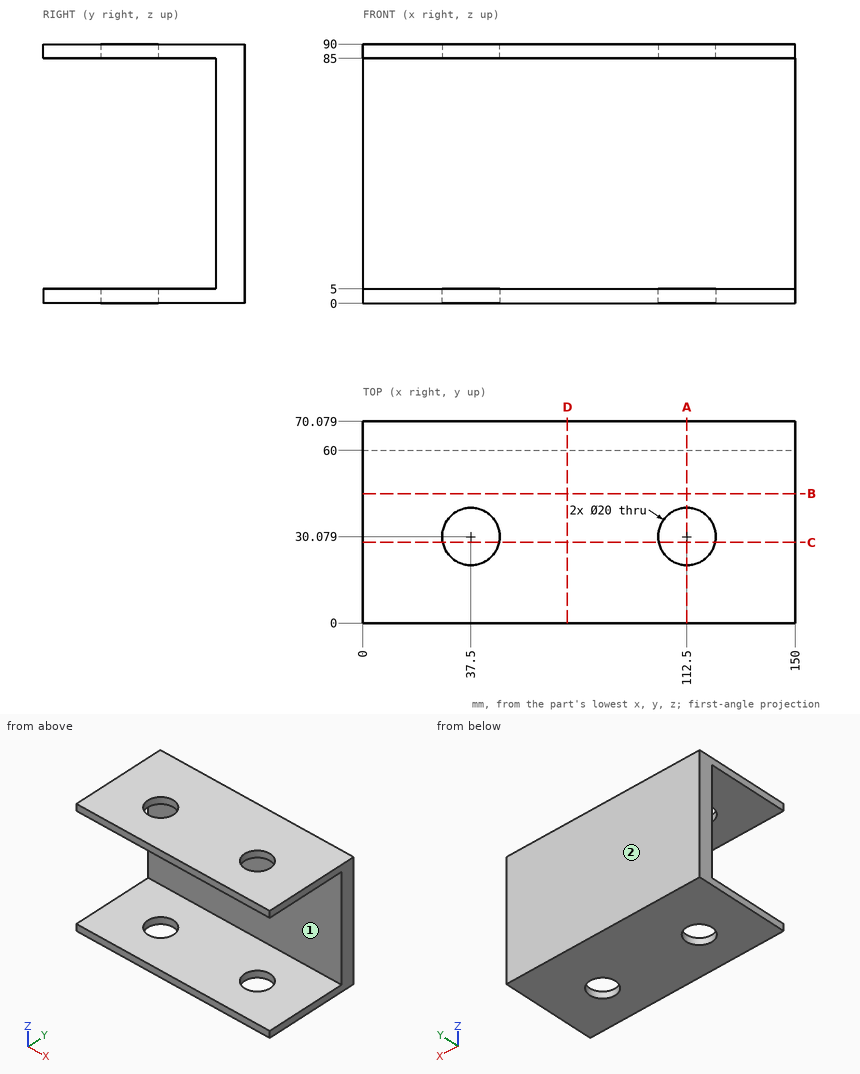
Geometry check sheet. Reference: drawing and pictorial views, mm from the part's lowest x, y, z. A direction names the side the tool comes from. Round coordinates to 2 decimals unless told otherwise and drop trailing zeros. Loops run counter-clockwise (first coordinate to the right, second up) from the corner with the lowest first, then second, coordinate; pieces in that order, holes last. Notation, with made-up numbers: (13.5, 45) - (38.5, 45) arc R30 ccw to (38.5, 73) - close; hole circle Ø9 at (-13.5, 66.5). An arc over 180 degrees is marked (long way). Answer in a Markdown table with one row per item. Add a question column.
Q1. Section check A-A on x = 112.5. Enter the section's corners in (y, z), plus the area to 3 significant figures.
Q2. Section check B-B on y = 45. Enter the section's corners in (x, z), plus the area to 3 significant figures.
Q3. Section check D-D on x = 71. Enter the section's corners in (y, z).
Q4. Section check C-C on y = 28. Enter the section's corners in (x, z).
Q5. Material ranges on line 1 (Z direction, x = 14, y = 7); line 2 (Y direction, x = 112, z = 2); line 3 (Y direction, x = 47.5, z = 74.5), recorded low to high.
Q6. Tool access check on the marked faces 1 and 2. Record the directions out of +Z, -Z, +X, -X, +Y, -Y that give a thin tool (end or side, any length) a straight path to the whole face; none if there is none.
Q7. Gauge pin test, flat ends, axial feed: pin 1 (1.5 mm diameter, centred on x = 61.5, z = 39.5, fed in from -Y); pin 2 (5 mm diameter, centred on x = 57.5, y = 33, fed in from -Z); pin 3 (16 mm diameter, centred on x = 112.5, y = 30.079, fed in from +Z). Record the tip position at first contact, or that the pin passes through.
Found:
| question | item | result |
|---|---|---|
| 1 | outline | (0, 0) - (20.08, 0) - (20.08, 5) - (0, 5) - close; (0, 85) - (20.08, 85) - (20.08, 90) - (0, 90) - close; (40.08, 0) - (70.08, 0) - (70.08, 90) - (40.08, 90) - (40.08, 85) - (60, 85) - (60, 5) - (40.08, 5) - close |
| 1 | area | 1,310 mm² |
| 2 | outline | (0, 0) - (150, 0) - (150, 5) - (0, 5) - close; (0, 85) - (150, 85) - (150, 90) - (0, 90) - close |
| 2 | area | 1,500 mm² |
| 3 | outline | (0, 0) - (70.08, 0) - (70.08, 90) - (0, 90) - (0, 85) - (60, 85) - (60, 5) - (0, 5) - close |
| 4 | outline | (0, 0) - (27.72, 0) - (27.72, 5) - (0, 5) - close; (0, 85) - (27.72, 85) - (27.72, 90) - (0, 90) - close; (47.28, 0) - (102.72, 0) - (102.72, 5) - (47.28, 5) - close; (47.28, 85) - (102.72, 85) - (102.72, 90) - (47.28, 90) - close; (122.28, 0) - (150, 0) - (150, 5) - (122.28, 5) - close; (122.28, 85) - (150, 85) - (150, 90) - (122.28, 90) - close |
| 5 | line 1 | z = 0 to 5, 85 to 90 |
| 5 | line 2 | y = 0 to 20.09, 40.07 to 70.08 |
| 5 | line 3 | y = 60 to 70.08 |
| 6 | face 1 | +X, -X, -Y |
| 6 | face 2 | +Z, -Z, +X, -X, +Y |
| 7 | pin 1 | stops at y = 60 |
| 7 | pin 2 | stops at z = 0 |
| 7 | pin 3 | passes through |
